Verification items for this drawing (mm, ordinates from the low corner). A direction names the side the tool comes from. Round coordinates to 2 decimals unless told otherwise and drop trailing zeros. Order: outer loops, then holes, each group sorted by start corner. A loop starts at its lowest first (then second) coordinate and runs counter-clockwise, first axis right, second up. Notation, with made-up numbers: (-40, 78.5) -> (-23, 78.5) arc R14 cw to (-23, 85.5) -> close; hole circle Ø6 at (45, 21.5). An arc over 180 degrees is marked (long way). Return JSON: item names as keys, results as strings. Group by question number.
Item 1: Access from +Z, -Z, +X, -X, +Y, -Y to the whole of each face (thin tool, end or side, straight path). Record for the marked faces 1, 2 and 3.
Item 2: Depth check by flat-ended pin: pin 1 Ø4.5 at (y, z) = (11.1, 19.1) entering from +X; pin 2 Ø3 at (x, z) = (11, 18) entering from +Y; pin 3 Ø5.5 at (y, z) = (11.1, 3.1) entering from -X. Enter the tip coordinate at first touch or a pass-through.
Item 3: Scan lines: probe 1 along Y at (x, z) = (6.75, 11.1); probe 2 along Z at (x, y) = (12.8, 19.1); probe 3 along Y at (x, z) = (7.75, 13.5). Record each from-to range of solid material in increasing order. Write a range as from..to.
Item 4: Draft check along Y on the marked faces 4, 5, 6 and 7. Enter one of: pulls with the +Y half, pulls with the -Y half, needs draft (parallel to the pull), parting line crosses it, or undercut.
Item 5: Sectioned sample at B-B on z = 3. Record the cut outline in (x, y).
Item 6: Sectioned sample at C-C on x = 13. Record the cut outline in (y, z).
Item 7: Sectioned sample at A-A on y = 11.1. Record the cut outline in (x, z), plus the area to 3 significant figures.
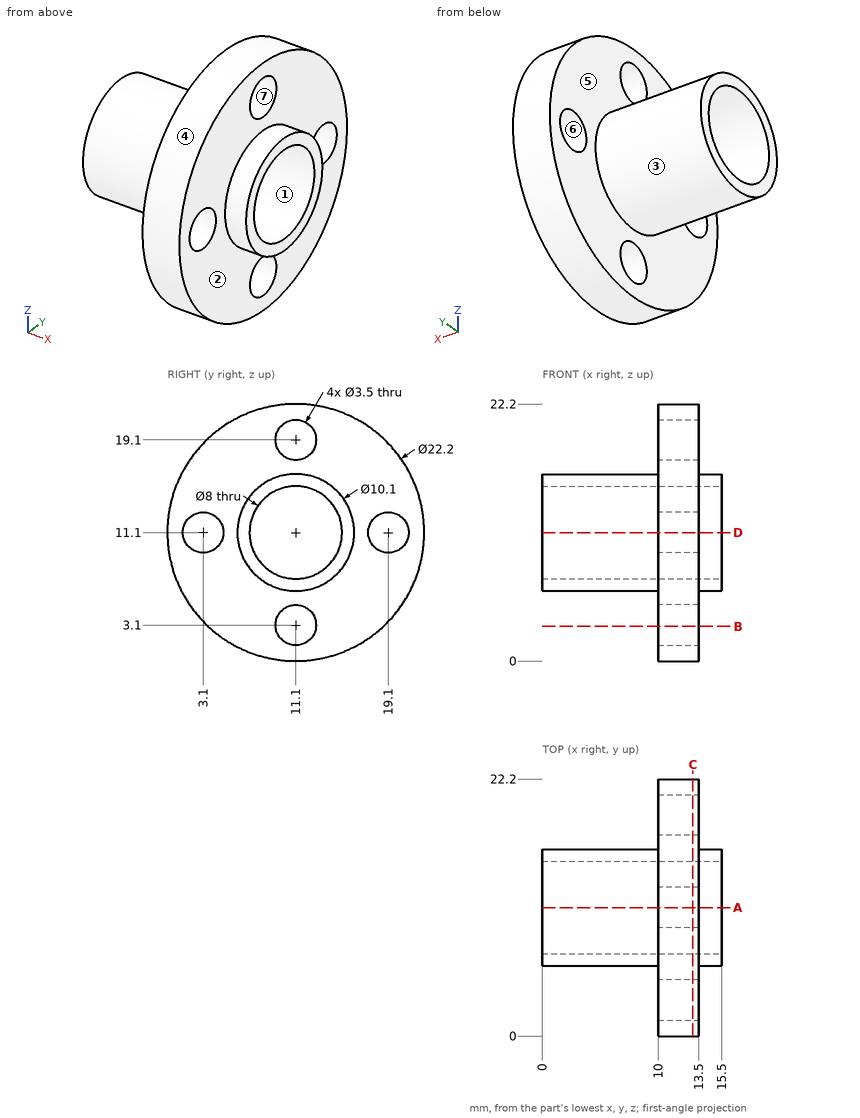
Recorded:
{
 "1": {"face 1": "+X, -X", "face 2": "+X", "face 3": "-X"},
 "2": {"pin 1": "x = 13.5", "pin 2": "y = 20.8", "pin 3": "x = 10"},
 "3": {"probe 1": "6.05..7.1, 15.1..16.15", "probe 2": "3.41..9.35, 12.85..18.79", "probe 3": "6.66..7.9, 14.3..15.54"},
 "4": {"face 4": "parting line crosses it", "face 5": "needs draft", "face 6": "undercut", "face 7": "undercut"},
 "5": {"outline": "(10, 3.51) -> (13.5, 3.51) -> (13.5, 9.35) -> (10, 9.35) -> close; (10, 12.85) -> (13.5, 12.85) -> (13.5, 18.69) -> (10, 18.69) -> close"},
 "6": {"outline": "circle Ø22.2 at (11.1, 11.1); hole circle Ø3.5 at (3.1, 11.1); hole circle Ø8 at (11.1, 11.1); hole circle Ø3.5 at (11.1, 3.1); hole circle Ø3.5 at (11.1, 19.1); hole circle Ø3.5 at (19.1, 11.1)"},
 "7": {"outline": "(0, 6.05) -> (10, 6.05) -> (10, 4.85) -> (13.5, 4.85) -> (13.5, 6.05) -> (15.5, 6.05) -> (15.5, 7.1) -> (0, 7.1) -> close; (0, 15.1) -> (15.5, 15.1) -> (15.5, 16.15) -> (13.5, 16.15) -> (13.5, 17.35) -> (10, 17.35) -> (10, 16.15) -> (0, 16.15) -> close; (10, 0) -> (13.5, 0) -> (13.5, 1.35) -> (10, 1.35) -> close; (10, 20.85) -> (13.5, 20.85) -> (13.5, 22.2) -> (10, 22.2) -> close", "area": "50.4 mm²"}
}
